CAD build for the part. Positions are in the model's coordinates, mm. Round coordinates to 2 decimals unless told otherwise and drop trailing zeros. Write each loop counter-clockwise with the first axis right and the second up, starting at its lowest first coordinate (ties: lowest second). Pieces come first, ordered by that corner, then holes. Notation, with made-up numbers: (73, -13.5) - (94, -13.5) arc R12 cw to (94, 2.5) - close; hole circle Ø2 at (-11, 56). An arc over 180 degrees is marked (long way). Answer in a Markdown table with one row per item.
```python
from build123d import *

# Parameters (mm, degrees)
SKETCH1_W                 = 6.35
SKETCH1_H                 = 37.666666667
SKETCH1_W_2               = 33.666666667
SKETCH1_H_2               = 6.35
BOSS_EXTRUDE1_DEPTH       = 3.175
MIRROR1_START             = -101
MIRROR1_OUTLINE_W         = 3.175
MIRROR1_OUTLINE_H         = 3.175
MIRROR1_OUTLINE_H_2       = 72.158333333
MIRROR1_DEPTH             = 101
MIRROR1_START_2           = -107.35
MIRROR1_2_OUTLINE_W       = 3.175
MIRROR1_2_OUTLINE_H       = 37.666666667
MIRROR1_2_DEPTH           = 70.508333333
MIRROR1_START_3           = -33.666666667
MIRROR1_3_OUTLINE_W       = 3.175
MIRROR1_3_OUTLINE_H       = 34.491666667
MIRROR1_3_OUTLINE_H_2     = 6.35
MIRROR1_3_DEPTH           = 33.666666667
MIRROR1_4_OUTLINE_W       = 3.175
MIRROR1_4_OUTLINE_H       = 3.175
MIRROR1_4_DEPTH           = 70.508333333
MIRROR4_COPY_1_SKETCH_W   = 6.35
MIRROR4_COPY_1_SKETCH_H   = 37.666666667
MIRROR4_COPY_1_SKETCH_W_2 = 33.666666667
MIRROR4_COPY_1_SKETCH_H_2 = 6.35
MIRROR4_COPY_1_DEPTH      = 3.175
MIRROR4_COPY_2_SKETCH_W   = 6.35
MIRROR4_COPY_2_SKETCH_H   = 37.666666667
MIRROR4_COPY_2_SKETCH_W_2 = 33.666666667
MIRROR4_COPY_2_SKETCH_H_2 = 6.35
MIRROR4_COPY_2_DEPTH      = 3.175


# Read off the part's stored shape, not the designer's step: Mirror1
with BuildPart() as part:
    # Sketch1 → Boss-Extrude1 (new body)
    with BuildSketch(Plane(origin=(0, 0, 0), x_dir=(1, 0, 0), z_dir=(0, 1, 0))):
        Polygon((-33.666666667, 113), (-101, 113), (-101, 37.666666667), (-101, 0), (-36.841666667, 0), (-36.841666667, 34.491666667), (-33.666666667, 34.491666667), (-33.666666667, 0), (0, 0), (0, 37.666666667), (-30.491666667, 37.666666667), (-30.491666667, 40.841666667), (0, 40.841666667), (0, 113), align=None)
        with Locations((-104.175, 18.833333334)):
            Rectangle(SKETCH1_W, SKETCH1_H)
        with Locations((-16.833333334, 116.175)):
            Rectangle(SKETCH1_W_2, SKETCH1_H_2)
    boss_extrude1 = extrude(amount=BOSS_EXTRUDE1_DEPTH)



with BuildPart() as body_2:
    # Mirror1 outline → Mirror1 (new body)
    with BuildSketch(Plane.YZ.offset(MIRROR1_START)):
        with Locations((1.5875, 36.079166667)):
            Rectangle(MIRROR1_OUTLINE_W, MIRROR1_OUTLINE_H)
        with Locations((1.5875, 76.920833333)):
            Rectangle(MIRROR1_OUTLINE_W, MIRROR1_OUTLINE_H_2)
    extrude(amount=MIRROR1_DEPTH)


with BuildPart() as part_1:
    add(part.part)

    add(body_2.part)  # Mirror1 2 merges body 2
    # Mirror1 2 outline → Mirror1 2 (add)
    with BuildSketch(Plane.YZ.offset(MIRROR1_START_2)):
        with Locations((1.5875, 18.833333334)):
            Rectangle(MIRROR1_2_OUTLINE_W, MIRROR1_2_OUTLINE_H)
    extrude(amount=MIRROR1_2_DEPTH)

    # Mirror1 3 outline → Mirror1 3 (add)
    with BuildSketch(Plane.YZ.offset(MIRROR1_START_3)):
        with Locations((1.5875, 17.245833334)):
            Rectangle(MIRROR1_3_OUTLINE_W, MIRROR1_3_OUTLINE_H)
        with Locations((1.5875, 116.175)):
            Rectangle(MIRROR1_3_OUTLINE_W, MIRROR1_3_OUTLINE_H_2)
    extrude(amount=MIRROR1_3_DEPTH)

    # Mirror1 4 outline → Mirror1 4 (add)
    with BuildSketch(Plane.YZ.offset(MIRROR1_START)):
        with Locations((1.5875, 39.254166667)):
            Rectangle(MIRROR1_4_OUTLINE_W, MIRROR1_4_OUTLINE_H)
    extrude(amount=MIRROR1_4_DEPTH)

    # Mirror3: Boss-Extrude1 across plane
    add(boss_extrude1.mirror(Plane(origin=(0, 0, 0), x_dir=(0, 0, 1), z_dir=(1, 0, 0))))

    # Mirror4 copy 1 sketch → Mirror4 copy 1 (add)
    with BuildSketch(Plane(origin=(0, 0, 0), x_dir=(-1, 0, 0), z_dir=(0, 1, 0))):
        Polygon((-33.666666667, 113), (-101, 113), (-101, 37.666666667), (-101, 0), (-36.841666667, 0), (-36.841666667, 34.491666667), (-33.666666667, 34.491666667), (-33.666666667, 0), (0, 0), (0, 37.666666667), (-30.491666667, 37.666666667), (-30.491666667, 40.841666667), (0, 40.841666667), (0, 113), align=None)
        with Locations((-104.175, 18.833333334)):
            Rectangle(MIRROR4_COPY_1_SKETCH_W, MIRROR4_COPY_1_SKETCH_H)
        with Locations((-16.833333334, 116.175)):
            Rectangle(MIRROR4_COPY_1_SKETCH_W_2, MIRROR4_COPY_1_SKETCH_H_2)
    extrude(amount=MIRROR4_COPY_1_DEPTH)

    # Mirror4 copy 2 sketch → Mirror4 copy 2 (add)
    with BuildSketch(Plane(origin=(0, 0, 0), x_dir=(1, 0, 0), z_dir=(0, 1, 0))):
        Polygon((-33.666666667, -113), (-101, -113), (-101, -37.666666667), (-101, 0), (-36.841666667, 0), (-36.841666667, -34.491666667), (-33.666666667, -34.491666667), (-33.666666667, 0), (0, 0), (0, -37.666666667), (-30.491666667, -37.666666667), (-30.491666667, -40.841666667), (0, -40.841666667), (0, -113), align=None)
        with Locations((-104.175, -18.833333334)):
            Rectangle(MIRROR4_COPY_2_SKETCH_W, MIRROR4_COPY_2_SKETCH_H)
        with Locations((-16.833333334, -116.175)):
            Rectangle(MIRROR4_COPY_2_SKETCH_W_2, MIRROR4_COPY_2_SKETCH_H_2)
    extrude(amount=MIRROR4_COPY_2_DEPTH)


solid = part_1.part
```
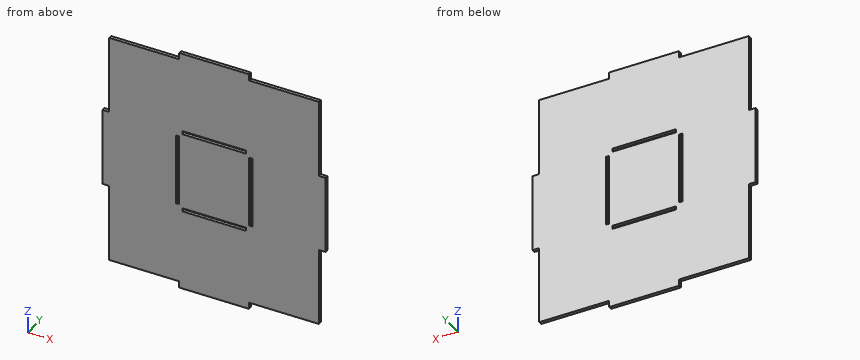
Q1. Saw through at D-D on x = -68.5. List the corners of the cut face in (y, z) (3 decimals).
Computed:
| item | result |
|---|---|
| outline | (0, -113) - (3.175, -113) - (3.175, 113) - (0, 113) - close |
Q2. Saw through at A-A on z = 5. List the corners of the cut face in (x, y) (3 decimals).
Computed:
| item | result |
|---|---|
| outline | (-107.35, 0) - (-36.842, 0) - (-36.842, 3.175) - (-107.35, 3.175) - close; (-33.667, 0) - (33.667, 0) - (33.667, 3.175) - (-33.667, 3.175) - close; (36.842, 0) - (107.35, 0) - (107.35, 3.175) - (36.842, 3.175) - close |
Q3. Drill centre lines: line 1 (Z direction, x = -9, y = 2.2); line 2 (X direction, y = 1.3, z = -12). Where is each one in solid material? Low to high.
Computed:
| item | result |
|---|---|
| line 1 | z = -119.35 to -40.84, -37.67 to 37.67, 40.84 to 119.35 |
| line 2 | x = -107.35 to -36.84, -33.67 to 33.67, 36.84 to 107.35 |
Q4. Flat gauge pins, fed straight in: pin 1 (12 mm diameter, centred on x = 59.5, z = 94, fed in from -Y); pin 2 (1 mm diameter, centred on y = 1, z = 115.5, fed in from -X); pin 3 (1.6 mm diameter, centred on y = 1, z = 39.5, fed in from +X); pin 4 (1.6 mm diameter, centred on y = 1, z = -38.5, fed in from -X). Where does each tip first touch, or does it go through?
Computed:
| item | result |
|---|---|
| pin 1 | stops at y = 0 |
| pin 2 | stops at x = -33.67 |
| pin 3 | stops at x = 101 |
| pin 4 | stops at x = -101 |
Q5. Saw through at B-B on x = 14. List the corners of the cut face in (y, z) (3 decimals).
Computed:
| item | result |
|---|---|
| outline | (0, -119.35) - (3.175, -119.35) - (3.175, -40.842) - (0, -40.842) - close; (0, -37.667) - (3.175, -37.667) - (3.175, 37.667) - (0, 37.667) - close; (0, 40.842) - (3.175, 40.842) - (3.175, 119.35) - (0, 119.35) - close |
Q6. Saw through at C-C on y = 2.1. Count the separate pieces of the cut face and the enclosed holes in it, then the cut area to 3 significant figures.
Computed:
| item | result |
|---|---|
| separate pieces | 1 |
| enclosed holes | 4 |
| area | 46,600 mm2 |
